from build123d import *

# Parameters (mm, degrees)
SKETCH_1_R          = 11.5
EXTRUDE_1_DEPTH     = 30
SKETCH_3_R          = 14.5
EXTRUDE_2_DEPTH     = 7
SKETCH_4_R          = 13.5
CUT_EXTRUDE_3_DEPTH = 5
CUT_EXTRUDE_START   = 1
SKETCH_2_R          = 10.5
CUT_EXTRUDE_2_DEPTH = 37


with BuildPart() as part:
    # ｽｹｯﾁ1 → ﾎﾞｽ - 押し出し1 (new body)
    with BuildSketch(Plane.XY):
        Circle(SKETCH_1_R)
    extrude(amount=EXTRUDE_1_DEPTH)

    # ｽｹｯﾁ3 → ﾎﾞｽ - 押し出し2 (add)
    with BuildSketch(Plane.XY.offset(30)):
        Circle(SKETCH_3_R)
    extrude(amount=EXTRUDE_2_DEPTH)

    # ｽｹｯﾁ4 → ｶｯﾄ - 押し出し3 (cut)
    with BuildSketch(Plane.XY.offset(37)):
        Circle(SKETCH_4_R)
    extrude(amount=-CUT_EXTRUDE_3_DEPTH, mode=Mode.SUBTRACT)

    # ｽｹｯﾁ2 → ｶｯﾄ - 押し出し2 (cut, through all)
    with BuildSketch(Plane.XY.offset(CUT_EXTRUDE_START)):
        Circle(SKETCH_2_R)
    extrude(amount=CUT_EXTRUDE_2_DEPTH, mode=Mode.SUBTRACT)


solid = part.part
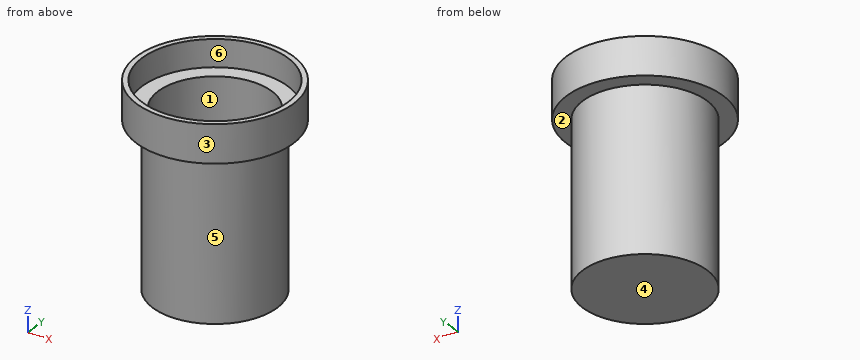
Design review of the part built by this model. Coordinates are the model's own, in mm. Face numbers are marked on the shaded views. A direction names the side the tool comes from. Round coordinates to 2 decimals unless told otherwise and drop trailing zeros. Write each loop counter-clockwise with the first axis right and the second up, starting at its lowest first coordinate (ties: lowest second). Pieces come first, ordered by that corner, then holes.
Item 1: Draft analysis for pull direction Y (two halves, no side actions). For the marked faces 1, 2 and 3, state which applies: released by +Y, released by -Y, zero draft, split by the parting line, or undercut.
Item 2: For pin 1 Ø17 at (x, y) = (0.5, -4.5) entering from +Z; pin 2 Ø2 at (y, z) = (9, 13) entering from +X; pin 3 Ø8 at (x, z) = (-6, 14) entering from -Y, all flat-tipped, find the tip position at first contact; note any pin that passes through.
Item 3: Wall thickness on L1, parallel to Y at x = 0, z = 33.8; L2, parallel to Y at x = 0, z = 23; L3, parallel to Z at x = -3, y = 4: over which ranges is each line inside the solid? List them lowest first.
Item 4: Consider section A-A on y = 0. Give the boundary of the cut face in (x, z).
Item 5: Consider section B-B on z = 30.5. Give the boundary of the cut face in (x, y), and give its area (3 significant figures).
Item 6: Consider section D-D on y = 12.75. Give the boundary of the cut face in (x, z).
Item 7: For the marked faces 4, 5 and 6, list the 3-axis set-ups (+Z, -Z, +X, -X, +Y, -Y) from which the entire face can be reached by the end or side of a thin tool; tool diameter is ignored.
Check values:
1. face 1: undercut
1. face 2: zero draft
1. face 3: split by the parting line
2. pin 1: stops at z = 32
2. pin 2: stops at x = 8.26
2. pin 3: stops at y = -11.32
3. L1: y = -14.5 to -13.5, 13.5 to 14.5
3. L2: y = -11.5 to -10.5, 10.5 to 11.5
3. L3: z = 0 to 1
4. outline: (-14.5, 30) - (-11.5, 30) - (-11.5, 0) - (11.5, 0) - (11.5, 30) - (14.5, 30) - (14.5, 37) - (13.5, 37) - (13.5, 32) - (10.5, 32) - (10.5, 1) - (-10.5, 1) - (-10.5, 32) - (-13.5, 32) - (-13.5, 37) - (-14.5, 37) - close
5. outline: circle Ø29 at (0, 0); hole circle Ø21 at (0, 0)
5. area: 314 mm2
6. outline: (-6.91, 30) - (6.91, 30) - (6.91, 37) - (4.44, 37) - (4.44, 32) - (-4.44, 32) - (-4.44, 37) - (-6.91, 37) - close
7. face 4: -Z, +X, -X, +Y, -Y
7. face 5: -Z
7. face 6: +Z
